Here's how the part is built. I have some questions about the finished solid (model axes, mm). A direction names the side the tool comes from. Give positions to 0.01 mm unless a question says otherwise; leave off trailing zeros. Loops run counter-clockwise (first coordinate to the right, second up) from the corner with the lowest first, then second, coordinate; pieces in that order, holes last.
Q1. Thinking about a two-plate mould opening in Y: for faces 1 (the face through (1.57, 11.12, 16.43)), 2 (the face through (2, 20, -98)), 3 (the face through (0, 20, -1)), which applies, pulls with the +Y half, pulls with the -Y half, needs draft (parallel to the pull), parting line crosses it, or undercut?
Q2. Suppose I cut it at B-B (x = 2.5). List the corners of the cut face in (y, z) for me (3 decimals), and give its area (3 significant figures).
Q3. I'm going to push flat-ended pins straight in: P1, Ø1.6, axis at x = 2, z = 99.5, coming from the -Y side; P2, Ø1, axis at x = 2, y = 12.5, coming from the -Z side; P3, Ø1, axis at x = 1, y = 18.5, coming from the -Z side; P4, Ø4.5, axis at y = 25, z = -95, coming from the -X side. Where does each tip first touch, or does it pass through?
Q4. I need wall thicknesses on probe 1 along Z at (x, y) = (0.8, 25) (3 decimals); probe 2 along Y at (x, z) = (0.7, -95); probe 3 along Z at (x, y) = (2.7, 15). Which ranges of each line are inside material? Lowest first, please.
Q5. Suppose I cut it at A-A (z = 95). List the corners of the cut face in (x, y) for me (3 decimals).
Q6. For faces 4 (the face through (2, 40, 1)), 5 (the face through (1.57, 28.88, 16.43)), 6 (the face through (2, 20, 98)), which set-ups out of +Z, -Z, +X, -X, +Y, -Y let a thin tool reach every point of the face, with its end or its side?
```python
from build123d import *

# Parameters (mm, degrees)
BOSS_EXTRUDE1_DEPTH                             = 3.175
CSK_FOR_M3_FLAT_HEAD_MACHINE_SCREW1_D           = 3.4
CSK_FOR_M3_FLAT_HEAD_MACHINE_SCREW1_CSINK_D     = 6.3
CSK_FOR_M3_FLAT_HEAD_MACHINE_SCREW1_CSINK_ANGLE = 90
CUT_EXTRUDE1_DEPTH                              = 4.175
FILLET1_R                                       = 3
FILLET1_OF_MIRROR3_R                            = 3


with BuildPart() as part:
    # Sketch1 → Boss-Extrude1 (new body)
    with BuildSketch(Plane(origin=(0, 0, 0), x_dir=(0, 0, -1), z_dir=(1, 0, 0))):
        with BuildLine():
            Line((-103.175, 20), (-103.175, 40))
            Line((-103.175, 40), (103.175, 40))
            Line((103.175, 40), (103.175, 20))
            Line((103.175, 20), (93, 20))
            ThreePointArc((93, 20), (90.878679656, 19.121320344), (90, 17))
            Line((90, 17), (90, 3))
            ThreePointArc((90, 3), (89.121320344, 0.878679656), (87, 0))
            Line((87, 0), (-87, 0))
            ThreePointArc((-87, 0), (-89.121320344, 0.878679656), (-90, 3))
            Line((-90, 3), (-90, 17))
            ThreePointArc((-90, 17), (-90.878679656, 19.121320344), (-93, 20))
            Line((-93, 20), (-103.175, 20))
        make_face()
    extrude(amount=BOSS_EXTRUDE1_DEPTH)

    # CSK for M3 Flat Head Machine Screw1 (through all)
    with Locations(Plane(origin=(3.175, 0, 0), x_dir=(0, 0, -1), z_dir=(1, 0, 0))):
        with Locations((-95, 25)):
            csk_for_m3_flat_head_machine_screw1 = CounterSinkHole(CSK_FOR_M3_FLAT_HEAD_MACHINE_SCREW1_D / 2, CSK_FOR_M3_FLAT_HEAD_MACHINE_SCREW1_CSINK_D / 2, counter_sink_angle=CSK_FOR_M3_FLAT_HEAD_MACHINE_SCREW1_CSINK_ANGLE)

    # Mirror1: CSK for M3 Flat Head Machine Screw1 across plane
    add(csk_for_m3_flat_head_machine_screw1.mirror(Plane.XY), mode=Mode.SUBTRACT)

    # Sketch4 → Cut-Extrude1 (cut, through all)
    with BuildSketch(Plane(origin=(3.175, 0, 0), x_dir=(0, 0, -1), z_dir=(1, 0, 0))):
        with BuildLine():
            Line((-15, 30), (-15, 10))
            ThreePointArc((-15, 10), (-25, 20), (-15, 30))
        make_face()
    cut_extrude1 = extrude(amount=-CUT_EXTRUDE1_DEPTH, mode=Mode.SUBTRACT)

    # Fillet1
    fillet1_edges = [part.edges().sort_by_distance(p)[0] for p in [
        (1.5875, 10, 15),
        (1.5875, 30, 15),
    ]]
    fillet(fillet1_edges, radius=FILLET1_R)

    # Mirror3: Cut-Extrude1 across plane
    add(cut_extrude1.mirror(Plane.XY), mode=Mode.SUBTRACT)

    # Fillet1 of Mirror3
    fillet1_of_mirror3_edges = [part.edges().sort_by_distance(p)[0] for p in [
        (1.5875, 10, -15),
        (1.5875, 30, -15),
    ]]
    fillet(fillet1_of_mirror3_edges, radius=FILLET1_OF_MIRROR3_R)


solid = part.part
```
Solutions:
1. face 1: undercut
1. face 2: pulls with the -Y half
1. face 3: needs draft
2. outline: (0, -87) arc R3 ccw to (3, -90) - (17, -90) arc R3 cw to (20, -93) - (20, -103.175) - (40, -103.175) - (40, 103.175) - (20, 103.175) - (20, 93) arc R3 cw to (17, 90) - (3, 90) arc R3 ccw to (0, 87) - close; hole (10.965, -19.286) arc R10 ccw to (29.035, -19.286) arc R3 ccw to (26.325, -15) - (13.675, -15) arc R3 ccw to start; hole (10.965, 19.286) arc R3 ccw to (13.675, 15) - (26.325, 15) arc R3 ccw to (29.035, 19.286) arc R10 ccw to start; hole circle Ø4.95 at (25, -95); hole circle Ø4.95 at (25, 95)
2. area: 7,390 mm2
3. P1: stops at y = 20
3. P2: stops at z = -90
3. P3: stops at z = -90.76
3. P4: stops at x = 0
4. probe 1: z = -103.175 to -96.7, -93.3 to -23.66, -15 to 15, 23.66 to 93.3, 96.7 to 103.175
4. probe 2: y = 20 to 23.3, 26.7 to 40
4. probe 3: z = -90 to -23.66, -15 to 15, 23.66 to 90
5. outline: (0, 20) - (3.175, 20) - (3.175, 21.85) - (1.725, 23.3) - (0, 23.3) - close; (0, 26.7) - (1.725, 26.7) - (3.175, 28.15) - (3.175, 40) - (0, 40) - close
6. face 4: +Z, -Z, +X, -X, +Y
6. face 5: +X, -X
6. face 6: +Z, +X, -X, -Y
